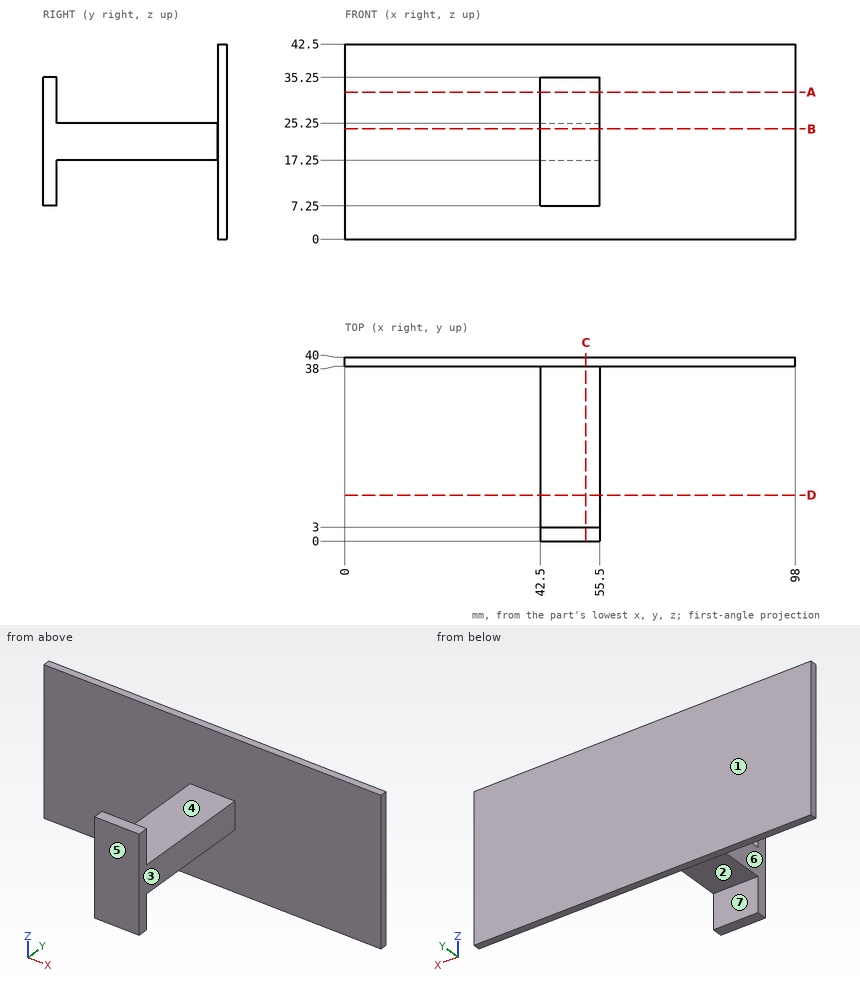
Answer from the drawing. Dimensions are ordinates in mm from the lowest x, y and z of the part. A direction names the side the tool comes from. Round coordinates to 2 decimals unless told otherwise and drop trailing zeros. Write each loop counter-clockwise with the first axis right and the second up, starting at its lowest first coordinate (ties: lowest second). Pieces come first, ordered by that corner, then holes. Notation, with made-up numbers: (-34.75, -2.75) -> (9.25, -2.75) arc R16 ccw to (9.25, 7.25) -> close; hole circle Ø8 at (54.5, 26.25). An arc over 180 degrees is marked (long way). Write each question's results on one line, items separated by ' | '.
1) For a pull along Y with two mould halves and no side action, classify the marked faces 4, 5, 6 and 7 as +Y half, -Y half, draft (parallel to the pull), parting line (faces both ways), or undercut.
Findings:
face 4: undercut | face 5: -Y half | face 6: draft | face 7: undercut
2) Flat-ended cylindrical pins translate along their axes: pin 1 (2.5 mm diameter, centred on x = 50.5, y = 2, fed in from -Z); pin 2 (1.5 mm diameter, centred on x = 82, z = 8, fed in from -Y); pin 3 (22.5 mm diameter, centred on y = 17, z = 25, fed in from -X); pin 4 (2 mm diameter, centred on x = 41, y = 7.5, fed in from +Z). Find the tip coordinate at first contact, or state that the pin passes through.
Findings:
pin 1: stops at z = 7.25 | pin 2: stops at y = 38 | pin 3: stops at x = 42.5 | pin 4: passes through
3) The part is cut by section B-B (z = 24). Write down the section's boundary in (x, y), and give its area (3 significant figures).
Findings:
outline: (0, 38) -> (42.5, 38) -> (42.5, 0) -> (55.5, 0) -> (55.5, 38) -> (98, 38) -> (98, 40) -> (0, 40) -> close | area: 690 mm²
4) Which of the six approach directions +Z, -Z, +X, -X, +Y, -Y give full straight-line access (tool end or side, diameter ignored) to the marked faces 1, 2 and 3?
Findings:
face 1: +Z, -Z, +X, -X, +Y | face 2: -Z, +X, -X | face 3: +Z, -Z, +X, -Y
5) Consider line 1 along Y through (x, z) = (75, 2); line 2 along Z through (x, y) = (47, 36.5); line 3 along Y through (x, z) = (50.5, 12). Determine where each line is inside the solid, lowest interval first. Write a range as [from, to].
Findings:
line 1: y = [38, 40] | line 2: z = [17.25, 25.25] | line 3: y = [0, 3], [38, 40]
6) The part is cut by section C-C (x = 52.5). Write down the section's boundary in (y, z), and give its area (3 significant figures).
Findings:
outline: (0, 7.25) -> (3, 7.25) -> (3, 17.25) -> (38, 17.25) -> (38, 0) -> (40, 0) -> (40, 42.5) -> (38, 42.5) -> (38, 25.25) -> (3, 25.25) -> (3, 35.25) -> (0, 35.25) -> close | area: 449 mm²
7) The part is cut by section A-A (z = 32). Write down the section's boundary in (x, y).
Findings:
outline: (0, 38) -> (98, 38) -> (98, 40) -> (0, 40) -> close; (42.5, 0) -> (55.5, 0) -> (55.5, 3) -> (42.5, 3) -> close
8) The part is cut by section D-D (y = 10). Write down the section's boundary in (x, z).
Findings:
outline: (42.5, 17.25) -> (55.5, 17.25) -> (55.5, 25.25) -> (42.5, 25.25) -> close
